The listing builds one solid part. Answer for the finished solid, in the listing's coordinates (mm). A direction names the side the tool comes from. Coordinates: 2 decimals unless noted, no trailing zeros. Order: outer loops, then holes, each group sorted by start corner. A loop starts at its lowest first (then second) coordinate and runs counter-clockwise, first axis right, second up. Notation, with made-up numbers: (-5.75, 62) -> (38.25, 62) arc R16 cw to (38.25, 87) -> close; hole circle Ø9 at (17, 80). An arc over 180 degrees is marked (long way). Return JSON: item names as keys, results as strings.
from build123d import *

# Parameters (mm, degrees)
SKETCH1_R           = 7.5
SKETCH1_W           = 8
SKETCH1_H           = 15
BOSS_EXTRUDE1_DEPTH = 10


with BuildPart() as part:
    # Sketch1 → Boss-Extrude1 (new body)
    with BuildSketch(Plane.XY):
        with BuildLine():
            Line((-79.357935679, -5.629473283), (-70.941049916, -42.048149016))
            ThreePointArc((-70.941049916, -42.048149016), (-69.113137448, -52.674804492), (-68.501205497, -63.440147491))
            Line((-68.501205497, -63.440147491), (-68.501205497, -93))
            ThreePointArc((-68.501205497, -93), (-67.036739403, -96.535533906), (-63.501205497, -98))
            Line((-63.501205497, -98), (-46.498794503, -98))
            ThreePointArc((-46.498794503, -98), (-42.963260597, -96.535533906), (-41.498794503, -93))
            Line((-41.498794503, -93), (-41.498794503, -63.440147491))
            ThreePointArc((-41.498794503, -63.440147491), (-40.886862552, -52.674804492), (-39.058950084, -42.048149016))
            Line((-39.058950084, -42.048149016), (-30.642064321, -5.629473283))
            ThreePointArc((-30.642064321, -5.629473283), (-55, 25), (-79.357935679, -5.629473283))
        make_face()
        with Locations((-55, 0)):
            Circle(SKETCH1_R, mode=Mode.SUBTRACT)
        with Locations((-55, -78)):
            Rectangle(SKETCH1_W, SKETCH1_H, mode=Mode.SUBTRACT)
    extrude(amount=BOSS_EXTRUDE1_DEPTH)


solid = part.part
1. Each of these flat-tipped pins is pushed along its axis until it touches: pin 1 Ø6 at (x, z) = (-47.5, 7) entering from +Y; pin 2 Ø2 at (y, z) = (-72.5, 2.5) entering from +X; pin 3 Ø1.5 at (x, z) = (-62.5, 6.5) entering from +Y. Where does it stop, or does it pass through?
Answer block:
{"pin 1": "stops at y = 24.59", "pin 2": "stops at x = -41.5", "pin 3": "stops at y = 24.07"}
2. The part is cut by section D-D on y = 0. Give the vertices of the cut face in (x, z), and give its area (3 significant figures).
Answer block:
{"outline": "(-80, 0) -> (-62.5, 0) -> (-62.5, 10) -> (-80, 10) -> close; (-47.5, 0) -> (-30, 0) -> (-30, 10) -> (-47.5, 10) -> close", "area": "350 mm2"}
3. Consider line 1 (Y direction, x = -55, z = 2); line 2 (X direction, y = -79, z = 6.5); line 3 (Y direction, x = -54, z = 5). Determine where each line is inside the solid, lowest interval first. Write a range as from..to.
Answer block:
{"line 1": "y = -98..-85.5, -70.5..-7.5, 7.5..25", "line 2": "x = -68.5..-59, -51..-41.5", "line 3": "y = -98..-85.5, -70.5..-7.43, 7.43..24.98"}
4. The part is cut by section C-C on z = 4.75. Give the vertices of the cut face in (x, y), and give its area (3 significant figures).
Answer block:
{"outline": "(-79.36, -5.63) -> (-70.94, -42.05) arc R95 cw to (-68.5, -63.44) -> (-68.5, -93) arc R5 ccw to (-63.5, -98) -> (-46.5, -98) arc R5 ccw to (-41.5, -93) -> (-41.5, -63.44) arc R95 cw to (-39.06, -42.05) -> (-30.64, -5.63) arc R25 ccw (long way) to start; hole circle Ø15 at (-55, 0); hole (-59, -85.5) -> (-51, -85.5) -> (-51, -70.5) -> (-59, -70.5) -> close", "area": "3,970 mm2"}
5. Determine the mould class of faces 4 (the face through (-41.499, -78, 5)), 5 (the face through (-55, -85.5, 5)), 6 (the face through (-67.075, -96.496, 4.93)) for opening direction Y: pulls with the +Y half, pulls with the -Y half, needs draft (parallel to the pull), parting line crosses it, or undercut.
Answer block:
{"face 4": "needs draft", "face 5": "undercut", "face 6": "pulls with the -Y half"}
6. The part is cut by section B-B on x = -55. Give the vertices of the cut face in (y, z).
Answer block:
{"outline": "(-98, 0) -> (-85.5, 0) -> (-85.5, 10) -> (-98, 10) -> close; (-70.5, 0) -> (-7.5, 0) -> (-7.5, 10) -> (-70.5, 10) -> close; (7.5, 0) -> (25, 0) -> (25, 10) -> (7.5, 10) -> close"}
7. For faces 1 (the face through (-34.91, -24.09, 4.93)), 2 (the face through (-68.501, -78, 5)), 3 (the face through (-59, -78, 5)), determine the directions among +Z, -Z, +X, -X, +Y, -Y from which every point of the face is accessible in a straight line to the end or side of a thin tool.
Answer block:
{"face 1": "+Z, -Z, +X, -Y", "face 2": "+Z, -Z, -X, -Y", "face 3": "+Z, -Z"}
8. The part is cut by section A-A on y = -83. Give the vertices of the cut face in (x, z).
Answer block:
{"outline": "(-68.5, 0) -> (-59, 0) -> (-59, 10) -> (-68.5, 10) -> close; (-51, 0) -> (-41.5, 0) -> (-41.5, 10) -> (-51, 10) -> close"}
